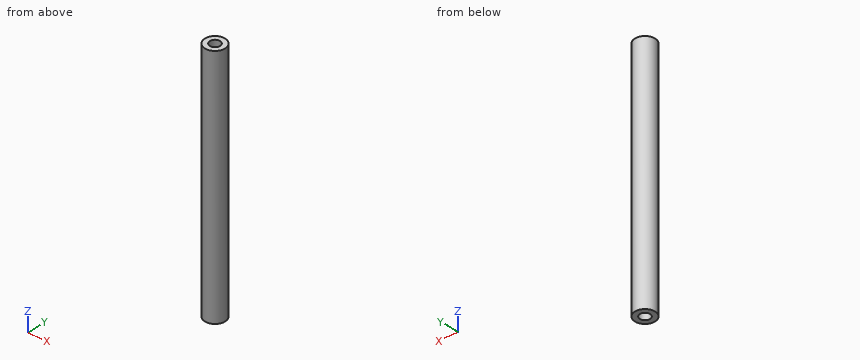
```python
from build123d import *

# Parameters (mm, degrees)
SKETCH1_R           = 10
BOSS_EXTRUDE1_DEPTH = 100
BOSS_EXTRUDE2_START = 20
SKETCH3_R           = 10
SKETCH3_R_2         = 5
BOSS_EXTRUDE2_DEPTH = 20


with BuildPart() as part:
    # Sketch1 → Boss-Extrude1 (new, symmetric)
    with BuildSketch(Plane.XY):
        Circle(SKETCH1_R)
    extrude(amount=BOSS_EXTRUDE1_DEPTH, both=True)

    # Sketch3 → Boss-Extrude2 (add)
    with BuildSketch(Plane.XY.offset(100).offset(BOSS_EXTRUDE2_START)):
        Circle(SKETCH3_R)
        Circle(SKETCH3_R_2, mode=Mode.SUBTRACT)
    boss_extrude2 = extrude(amount=-BOSS_EXTRUDE2_DEPTH)

    # Mirror1: Boss-Extrude2 across plane
    add(boss_extrude2.mirror(Plane.XY))


solid = part.part
```
The model under review builds one solid part; all positions refer to its coordinate system, in mm. Coordinates: 2 decimals unless noted, no trailing zeros. Loops run counter-clockwise (first coordinate to the right, second up) from the corner with the lowest first, then second, coordinate; pieces in that order, holes last. Notation, with made-up numbers: (27.25, -20.75) -> (73.25, -20.75) arc R11 ccw to (73.25, -3.75) -> close; hole circle Ø3 at (-21, 35.5). An arc over 180 degrees is marked (long way). Answer as CSV lines item,"result".
Item 1: Take a section at B-B, the plane z = 45.5. State the section outline as (x, y) points, and give its area (3 significant figures).
Results below:
outline,"circle Ø20 at (0, 0)"
area,"314 mm2"
Item 2: Take a section at A-A, the plane x = 0. State the section outline as (y, z) points, and give its area (3 significant figures).
Results below:
outline,"(-10, -120) -> (-5, -120) -> (-5, -100) -> (5, -100) -> (5, -120) -> (10, -120) -> (10, 120) -> (5, 120) -> (5, 100) -> (-5, 100) -> (-5, 120) -> (-10, 120) -> close"
area,"4,400 mm2"
Item 3: For L1, parallel to Y at x = 0, z = -114; L2, parallel to Z at x = -3.5, y = 1; L3, parallel to X at y = 1.5, z = 45.5, list the stretches that pass through material, from the lowest coordinate up.
Results below:
L1,"y = -10 to -5, 5 to 10"
L2,"z = -100 to 100"
L3,"x = -9.89 to 9.89"
Item 4: Insertion check: pin 1 (10 mm diameter, centred on y = 7.5, z = -10.5, fed in from -X); pin 2 (4 mm diameter, centred on x = -7, z = 92.5, fed in from -Y); pin 3 (3 mm diameter, centred on x = -1, y = 0.5, fed in from +Z). Each pin has a flat end and moves straight along its axis. Give the tip position at first contact, or say it passes through.
Results below:
pin 1,"stops at x = -9.68"
pin 2,"stops at y = -8.66"
pin 3,"stops at z = 100"
